```python
from build123d import *

# Parameters (mm, degrees)
SKETCH1_R           = 2.5
BOSS_EXTRUDE1_DEPTH = 0.5
SKETCH2_R           = 1.5
SKETCH2_R_2         = 1
BOSS_EXTRUDE2_DEPTH = 5


with BuildPart() as part:
    # Sketch1 → Boss-Extrude1 (new body)
    with BuildSketch(Plane(origin=(0, 0, 0), x_dir=(1, 0, 0), z_dir=(0, 1, 0))):
        with BuildLine():
            Line((0, -1), (0, 1))
            Line((0, 1), (1.5, 1))
            ThreePointArc((1.5, 1), (10.286184959, 0), (1.5, -1))
            Line((1.5, -1), (0, -1))
        make_face()
        with Locations((5.836184959, 0)):
            Circle(SKETCH1_R, mode=Mode.SUBTRACT)
    extrude(amount=BOSS_EXTRUDE1_DEPTH)

    # Sketch2 → Boss-Extrude2 (add)
    with BuildSketch(Plane(origin=(0.5, 0.5, 0), x_dir=(0, 0, -1), z_dir=(0, 1, 0))):
        with Locations((0, 0.5)):
            Circle(SKETCH2_R)
        with Locations((0, 0.5)):
            Circle(SKETCH2_R_2, mode=Mode.SUBTRACT)
    extrude(amount=-BOSS_EXTRUDE2_DEPTH)


solid = part.part
```
Geometry check sheet. Reference: the model listing, model coordinates, mm. A direction names the side the tool comes from. Round coordinates to 2 decimals unless told otherwise and drop trailing zeros. Order: outer loops, then holes, each group sorted by start corner. A loop starts at its lowest first (then second) coordinate and runs counter-clockwise, first axis right, second up. Notation, with made-up numbers: (10.25, -16) -> (25.25, -16) arc R17 ccw to (25.25, -1) -> close; hole circle Ø2 at (-21.75, -15). An arc over 180 degrees is marked (long way). Return JSON: item names as keys, results as strings. Group by question number.
Q1. Gauge pin test, flat ends, axial feed: pin 1 (1 mm diameter, centred on x = 7.5, z = 1.5, fed in from -Y); pin 2 (2 mm diameter, centred on y = -1, z = 1, fed in from -X); pin 3 (3 mm diameter, centred on x = 2.5, y = -3.5, fed in from +Z). Record the tip position at first contact, or that the pin passes through.
Q2. Section check C-C, the plane y = -3.3. Record the boundary of the cut face in (x, z).
Q3. Section check B-B, the plane x = 3.5. Record the boundary of the cut face in (y, z).
Q4. Release check for a two-part mould opening along Z. For faces 3 (the cylindrical face through (3.34, 0.25, -0.11)), 4 (the cylindrical face through (-1, -2, 0)), 5 (the cylindrical face through (10.282, 0.246, -0.182)), 6 (the flat face through (8, 0, 2)) record: released by +Z, released by -Z, zero draft, split by the parting line, or undercut.
Q5. Section check A-A, the plane z = 0. Record the boundary of the cut face in (x, y).
Q6. Material ranges on probe 1 along X at (y, z) = (0.35, 0); probe 2 along X at (y, z) = (-2.6, 0); probe 3 along Y at (x, z) = (1.75, -0.5), recorded low to high. Write a range as from..to.
Q7. Tool access check on faces 1 (the cylindrical face through (-1.487, -1.965, 0.195)), 2 (the flat face through (3, 0.5, 0)). Record the directions out of +Z, -Z, +X, -X, +Y, -Y that give a thin tool (end or side, any length) a straight path to the whole face; none if there is none.
Q8. Section check D-D, the plane x = 6.75. Record the boundary of the cut face in (y, z), plus the area to 3 significant figures.
Numbers:
{
 "1": {"pin 1": "y = 0", "pin 2": "x = -1.5", "pin 3": "z = 1.12"},
 "2": {"outline": "circle Ø3 at (0, 0); hole circle Ø2 at (0, 0)"},
 "3": {"outline": "(0, -3.79) -> (0.5, -3.79) -> (0.5, -0.89) -> (0, -0.89) -> close; (0, 0.89) -> (0.5, 0.89) -> (0.5, 3.79) -> (0, 3.79) -> close"},
 "4": {"face 3": "undercut", "face 4": "undercut", "face 5": "split by the parting line", "face 6": "zero draft"},
 "5": {"outline": "(-1.5, -4.5) -> (-1, -4.5) -> (-1, 0.5) -> (-1.5, 0.5) -> close; (0, 0) -> (1, 0) -> (1, -4.5) -> (1.5, -4.5) -> (1.5, 0) -> (3.34, 0) -> (3.34, 0.5) -> (0, 0.5) -> close; (8.34, 0) -> (10.29, 0) -> (10.29, 0.5) -> (8.34, 0.5) -> close"},
 "6": {"probe 1": "-1.5..-1, 0..3.34, 8.34..10.29", "probe 2": "-1.5..-1, 1..1.5", "probe 3": "0..0.5"},
 "7": {"face 1": "-Y", "face 2": "+Z, -Z, +X, -X, +Y"},
 "8": {"outline": "(0, -4.36) -> (0.5, -4.36) -> (0.5, -2.33) -> (0, -2.33) -> close; (0, 2.33) -> (0.5, 2.33) -> (0.5, 4.36) -> (0, 4.36) -> close", "area": "2.03 mm^2"}
}
